Build history of the part. All positions in model axes, mm. A direction names the side the tool comes from. Round coordinates to 2 decimals unless told otherwise and drop trailing zeros. Write each loop counter-clockwise with the first axis right and the second up, starting at its lowest first coordinate (ties: lowest second). Pieces come first, ordered by that corner, then holes.
Item 1: Wall check: probe 1 along Z at (x, y) = (-3, 1.75); probe 2 along Y at (x, z) = (0, 6.25); probe 3 along Y at (x, z) = (-0.5, 9.5). Give the ranges that are in metal, low to high.
Item 2: Band-saw the part on A-A, the plane x = 0.25. Write the cut outline in (y, z).
Item 3: 3-axis set-ups, long thin cutter, end or side, ignore diameter. For faces 1 (the cylindrical face through (0, 2, 5)), 2 (the flat face through (0, 0, 0)), 3 (the flat face through (1, 0, 10)): which of +Z, -Z, +X, -X, +Y, -Y reach the whole face in a straight line?
Item 4: Mould opens along X. For faces 4 (the flat face through (1, -1, 11.5)), 5 (the flat face through (-0.51, 0.86, 10.27)), 6 (the cylindrical face through (-0.867, 3.905, 10.74)) say: +X half, -X half, draft (parallel to the pull), parting line (faces both ways), or undercut.
Item 5: Band-saw the part on B-B, the plane y = 0. Write the cut outline in (x, z), then the cut area to 3 significant figures.
Item 6: Band-saw the part on D-D, the plane x = 1.5. Write the cut outline in (y, z).
Item 7: Drop flat-ended pins along their axis: pin 1 Ø3 at (y, z) = (-2.5, 10.5) entering from -X; pin 2 Ø3 at (x, z) = (3, 4) entering from -Y; pin 3 Ø1.5 at (y, z) = (2, 5) entering from -X. Give the stop position or say it passes through.
Item 8: Band-saw the part on C-C, the plane z = 8.5. Write the cut outline in (x, y), then the cut area to 3 significant figures.
Autodesk Inventor part; units mm, degrees
ref_plane "YZ Plane" through (0, 0, 0) normal (1, 0, 0) x (0, 1, 0)
ref_plane "XZ Plane" through (0, 0, 0) normal (0, 1, 0) x (-1, 0, 0)
ref_plane "XY Plane" through (0, 0, 0) normal (0, 0, 1) x (1, 0, 0)
sketch "スケッチ1" plane through (0, 0, 0) normal (0, 0, 1) x (1, 0, 0)
  circle A0 centre (0, 0) radius 2
  dimension "d0" = 4
extrude "押し出し1" add sketch "スケッチ1" along normal blind 10
thread "ねじ1"
sketch "スケッチ2" plane through (0, 0, 10) normal (0, 0, 1) x (1, 0, 0)
  circle A0 centre (0, 0) radius 4
  dimension "d5" = 8
extrude "押し出し2" add sketch "スケッチ2" along normal blind 1.5
sketch "スケッチ3" plane through (0, 0, 11.5) normal (0, 0, 1) x (1, 0, 0)
  line L0 (0, 1.1547) -> (1, 0.5774)
  line L1 (1, 0.5774) -> (1, -0.5774)
  line L2 (1, -0.5774) -> (0, -1.1547)
  line L3 (0, -1.1547) -> (-1, -0.5774)
  line L4 (-1, -0.5774) -> (-1, 0.5774)
  line L5 (-1, 0.5774) -> (0, 1.1547)
  point P0 (0, 0)
  point P1 (0, 0)
  dimension "d8" = 2
extrude "押し出し3" cut sketch "スケッチ3" against normal blind 2.5
properties part number "M4極低頭ネジ　10" material "鋼、高強度、低合金"
Results:
1. probe 1: z = 10 to 11.5
1. probe 2: y = -2 to 2
1. probe 3: y = -1.94 to -0.87, 0.87 to 1.94
2. outline: (-3.99, 10) - (-1.98, 10) - (-1.98, 0) - (1.98, 0) - (1.98, 10) - (3.99, 10) - (3.99, 11.5) - (1.01, 11.5) - (1.01, 9) - (-1.01, 9) - (-1.01, 11.5) - (-3.99, 11.5) - close
3. face 1: -Z
3. face 2: -Z, +X, -X, +Y, -Y
3. face 3: +Z
4. face 4: draft
4. face 5: undercut
4. face 6: parting line
5. outline: (-4, 10) - (-2, 10) - (-2, 0) - (2, 0) - (2, 10) - (4, 10) - (4, 11.5) - (1, 11.5) - (1, 9) - (-1, 9) - (-1, 11.5) - (-4, 11.5) - close
5. area: 47.0 mm2
6. outline: (-3.71, 10) - (-1.32, 10) - (-1.32, 0) - (1.32, 0) - (1.32, 10) - (3.71, 10) - (3.71, 11.5) - (-3.71, 11.5) - close
7. pin 1: stops at x = -3.87
7. pin 2: stops at y = -1.32
7. pin 3: stops at x = -1.56
8. outline: circle Ø4 at (0, 0)
8. area: 12.6 mm2
